```python
from build123d import *

# Parameters (mm, degrees)
SKETCH1_R      = 1.395
EXTRUDE1_DEPTH = 4.955
SKETCH2_W      = 9.906
SKETCH2_H      = 0.508
EXTRUDE2_DEPTH = 3.105
EXTRUDE3_DEPTH = 2.415
EXTRUDE4_DEPTH = 2.92
EXTRUDE5_REACH = 29.791
SKETCH5_W      = 6.351205797
SKETCH5_H      = 0.762
SKETCH5_H_2    = 0.76
EXTRUDE6_REACH = 29.791
SKETCH_R       = 0.762
FILLET1_R      = 0.508
SKETCH6_R      = 0.635
EXTRUDE7_DEPTH = 4.572
SKETCH_2_R     = 1.395
EXTRUDE8_DEPTH = 7.92


with BuildPart() as part:
    # Sketch1 → Extrude1 (new body, symmetric)
    with BuildSketch(Plane.XY):
        with Locations((-11.3, 5.08)):
            Circle(SKETCH1_R)
        with BuildLine():
            Line((13.97, -5.334), (13.97, 5.334))
            ThreePointArc((13.97, 5.334), (13.226051224, 7.130051224), (11.43, 7.874))
            Line((11.43, 7.874), (-11.43, 7.874))
            ThreePointArc((-11.43, 7.874), (-13.226051224, 7.130051224), (-13.97, 5.334))
            Line((-13.97, 5.334), (-13.97, 3.048))
            Line((-13.97, 3.048), (-14.732, 3.048))
            Line((-14.732, 3.048), (-14.732, -4.572))
            Line((-14.732, -4.572), (-13.97, -4.572))
            Line((-13.97, -4.572), (-13.97, -5.334))
            ThreePointArc((-13.97, -5.334), (-13.226051224, -7.130051224), (-11.43, -7.874))
            Line((-11.43, -7.874), (11.43, -7.874))
            ThreePointArc((11.43, -7.874), (13.226051224, -7.130051224), (13.97, -5.334))
        make_face()
        with Locations((11.3, -5.16)):
            Circle(SKETCH1_R, mode=Mode.SUBTRACT)
        with Locations((-11.3, 5.08)):
            Circle(SKETCH1_R, mode=Mode.SUBTRACT)
        with Locations((11.3, -5.16)):
            Circle(SKETCH1_R)
    extrude(amount=EXTRUDE1_DEPTH, both=True)

    # Sketch2 → Extrude2 (add, symmetric)
    with BuildSketch(Plane.XY):
        with Locations((-19.685, -2.54)):
            Rectangle(SKETCH2_W, SKETCH2_H)
        with Locations((-19.685, 1.524)):
            Rectangle(SKETCH2_W, SKETCH2_H)
    extrude(amount=EXTRUDE2_DEPTH, both=True)

    # Sketch3 → Extrude3 (add, symmetric)
    with BuildSketch(Plane.XY):
        Polygon((47.128347754, 14.344963285), (-3.048, 9.862642591), (-3.048, 7.874), (-2.54, 7.874), (-2.54, 9.398), (47.173548085, 13.838978176), align=None)
        with BuildLine():
            Line((10.16, 7.874), (10.16, 9.139))
            ThreePointArc((10.16, 9.139), (8.89, 10.409), (7.62, 9.139))
            Line((7.62, 9.139), (7.62, 7.874))
            Line((7.62, 7.874), (10.16, 7.874))
        make_face()
    extrude(amount=EXTRUDE3_DEPTH, both=True)

    # Sketch4 → Extrude4 (add, symmetric)
    with BuildSketch(Plane.XY):
        Polygon((-0.38, -10.984), (-0.38, -7.874), (-1.015, -7.874), (-1.015, -10.414), (-10.612457197, -11.452431876), (-10.54414973, -12.083747241), align=None)
    extrude(amount=EXTRUDE4_DEPTH, both=True)

    # Sketch5 → Extrude5 (cut, up to next)
    with BuildSketch(Plane(origin=(1.170304596, -10.816259141, 0), x_dir=(0.994197425, 0.107570815, 0), z_dir=(0.107570815, -0.994197425, 0)), mode=Mode.PRIVATE) as extrude5_sk1:
        with Locations((-8.607222155, 2.539)):
            Rectangle(SKETCH5_W, SKETCH5_H)
    extrude5_tool1 = extrude(extrude5_sk1.sketch, amount=-EXTRUDE5_REACH, mode=Mode.PRIVATE) & part.part
    add(extrude5_tool1.solids().sort_by_distance((-7.386974, -11.742145, 2.539))[0], mode=Mode.SUBTRACT)
    # Sketch5 → Extrude5 (cut, up to next)
    with BuildSketch(Plane(origin=(1.170304596, -10.816259141, 0), x_dir=(0.994197425, 0.107570815, 0), z_dir=(0.107570815, -0.994197425, 0)), mode=Mode.PRIVATE) as extrude5_sk2:
        with Locations((-8.607222155, -2.54)):
            Rectangle(SKETCH5_W, SKETCH5_H_2)
    extrude5_tool2 = extrude(extrude5_sk2.sketch, amount=-EXTRUDE5_REACH, mode=Mode.PRIVATE) & part.part
    add(extrude5_tool2.solids().sort_by_distance((-7.386974, -11.742145, -2.54))[0], mode=Mode.SUBTRACT)

    # Sketch → Extrude6 (cut, up to next)
    with BuildSketch(Plane(origin=(1.170304596, -10.816259141, 0), x_dir=(0.994197425, 0.107570815, 0), z_dir=(0.107570815, -0.994197425, 0)), mode=Mode.PRIVATE) as extrude6_sk1:
        with Locations((-8.101824296, 0)):
            Circle(SKETCH_R)
    extrude6_tool1 = extrude(extrude6_sk1.sketch, amount=-EXTRUDE6_REACH, mode=Mode.PRIVATE) & part.part
    add(extrude6_tool1.solids().sort_by_distance((-6.884508, -11.687779, 0))[0], mode=Mode.SUBTRACT)

    # Fillet1
    fillet1_edges = [part.edges().sort_by_distance(p)[0] for p in [
        (-4.263951014, -11.084885172, 2.92),
        (-10.578303464, -11.768089558, 2.158),
        (-10.578303464, -11.768089558, -2.16),
        (-4.263951014, -11.084885172, -2.92),
        (-3.048, 9.862642591, 0),
        (-2.54, 9.398, 0),
        (-0.38, -10.984, 0),
        (-1.015, -10.414, 0),
    ]]
    fillet(fillet1_edges, radius=FILLET1_R)

    # Sketch6 → Extrude7 (cut)
    with BuildSketch(Plane.XZ.offset(2.794)):
        with Locations((-21.462, 0)):
            Circle(SKETCH6_R)
    extrude(amount=-EXTRUDE7_DEPTH, mode=Mode.SUBTRACT)

    # Sketch 2 → Extrude8 (cut, symmetric)
    with BuildSketch(Plane.XY):
        with Locations((-11.3, 5.08)):
            Circle(SKETCH_2_R)
        with Locations((11.3, -5.16)):
            Circle(SKETCH_2_R)
    extrude(amount=EXTRUDE8_DEPTH, both=True, mode=Mode.SUBTRACT)


solid = part.part
```
Model file for the job. Use its own axes, mm. A direction names the side the tool comes from. Coordinates: 2 decimals unless noted, no trailing zeros. Order: outer loops, then holes, each group sorted by start corner. A loop starts at its lowest first (then second) coordinate and runs counter-clockwise, first axis right, second up. Notation, with made-up numbers: M 22.25,-23 L 58.25,-23 A10 cw 58.25,-19 Z; hole C 70,-27 d8. An arc over 180 degrees is marked long. Answer as CSV lines item,"result".
(1) Flat gauge pins, fed straight in: pin 1 (0.6 mm diameter, centred on x = -18, y = 1.5, fed in from +Z) (3 decimals); pin 2 (1.9 mm diameter, centred on x = 33.5, y = 12, fed in from +Z) (3 decimals); pin 3 (2 mm diameter, centred on x = -21.462, z = 0, fed in from +Y); pin 4 (1.7 mm diameter, centred on x = -11.3, y = 5.08, fed in from +Z). Where does each tip first touch, or does it go through?
Geometry says:
pin 1,"stops at z = 3.105"
pin 2,"stops at z = 2.415"
pin 3,"stops at y = 1.78"
pin 4,"passes through"
(2) 3-axis set-ups, long thin cutter, end or side, ignore diameter. For faces 5 (the flat face through (9, 9, 2.415)), 6 (the cylindrical face through (13.246, 7.11, 0.069)), 7 (the flat face through (9, 9, -2.415)), 8 (the flat face through (-0.38, -9, 0)), 9 (the flat face through (-1.015, -9, 0)): which of +Z, -Z, +X, -X, +Y, -Y reach the whole face in a straight line?
Geometry says:
face 5,"+Z, +X, -X, +Y"
face 6,"+Z, -Z, +X"
face 7,"-Z, +X, -X, +Y"
face 8,"+Z, -Z, +X, -Y"
face 9,"+Z, -Z, -X"
(3) Band-saw the part on B-B, the plane z = 0. State how many separate pieces and enclosed holes the cut face has, then the cut area to 3 significant figures.
Geometry says:
separate pieces,"4"
enclosed holes,"2"
area,"476 mm2"
(4) Band-saw the part on D-D, the plane x = 35. List the corners of the cut face in (y, z) (1 decimal).
Geometry says:
outline,"M 12.8,-2.4 L 13.3,-2.4 L 13.3,2.4 L 12.8,2.4 Z"
(5) Pull direction Y, two halves, no side cores. Call faces 1 (the flat face through (7.62, 8.5, 0)), 2 (the cylindrical face through (-13.246, -7.11, 0.069)), 3 (the flat face through (-20, 1.27, 0)), 4 (the flat face through (-1, 0, 4.955)): +Y half, -Y half, draft (parallel to the pull), parting line (faces both ways), or undercut.
Geometry says:
face 1,"undercut"
face 2,"-Y half"
face 3,"undercut"
face 4,"draft"
(6) Band-saw the part on A-A, the plane x = 3. List the corners of the cut face in (y, z) (3 decimals), then the cut area to 3 significant figures.
Geometry says:
outline,"M -7.874,-4.955 L 7.874,-4.955 L 7.874,4.955 L -7.874,4.955 Z; M 9.893,-2.415 L 10.403,-2.415 L 10.403,2.415 L 9.893,2.415 Z"
area,"159 mm2"
(7) Wall check: line 1 along Y through (x, z) = (-11.3, 1.75) (3 decimals); line 2 along Y through (x, z) = (-16, 2); line 3 along Y through (x, z) = (11.3, -0.5) (3 decimals). Give the ranges that are in metal, low to high.
Geometry says:
line 1,"y = -7.874 to 3.685, 6.475 to 7.874"
line 2,"y = -2.79 to -2.29, 1.27 to 1.78"
line 3,"y = -7.874 to -6.555, -3.765 to 7.874, 10.634 to 11.144"
(8) Band-saw the part on C-C, the plane y = 11.5. List the corners of the cut face in (x, z) (3 decimals), then the cut area to 3 significant figures.
Geometry says:
outline,"M 15.281,-2.415 L 20.99,-2.415 L 20.99,2.415 L 15.281,2.415 Z"
area,"27.6 mm2"
